```python
from build123d import *

# Parameters (mm, degrees)
SKETCH1_W                      = 6
SKETCH1_H                      = 27
BOSS_EXTRUDE1_DEPTH            = 5
BOSS_EXTRUDE2_START            = 5
BOSS_EXTRUDE2_DEPTH            = 55
CHAMFER1_SIZE                  = 20
CHAMFER1_SIZE_2                = 27.527638409
M3_CLEARANCE_HOLE1_D           = 3.6
M3_CLEARANCE_HOLE1_CSINK_D     = 3.65
M3_CLEARANCE_HOLE1_CSINK_ANGLE = 90
CUT_EXTRUDE1_DEPTH             = 70.865943062
CUT_EXTRUDE1_DEPTH_BACK        = 70.865943062
SKETCH4_R                      = 6.5
F_5_3_5_3_DIAMETER_HOLE1_D     = 5.3
F_5_3_5_3_DIAMETER_HOLE1_DEPTH = 7
F_5_3_5_3_DIAMETER_HOLE1_TIP   = 1.59228064
SKETCH10_R                     = 3
CUT_EXTRUDE2_DEPTH             = 10
SKETCH11_R                     = 2.5
CUT_EXTRUDE3_DEPTH             = 81.857900047


with BuildPart() as part:
    # Sketch1 → Boss-Extrude1 (new body)
    with BuildSketch(Plane(origin=(0, 0, 0), x_dir=(1, 0, 0), z_dir=(0, 1, 0))):
        with Locations((-20.5, -13.5)):
            Rectangle(SKETCH1_W, SKETCH1_H)
        Polygon((-23.5, 0), (-17.5, 0), (17.5, 0), (23.5, 0), (23.5, 6), (-23.5, 6), align=None)
        with Locations((20.5, -13.5)):
            Rectangle(SKETCH1_W, SKETCH1_H)
    extrude(amount=BOSS_EXTRUDE1_DEPTH)

    # Sketch1<3> → Boss-Extrude2 (add)
    with BuildSketch(Plane(origin=(0, 0, 0), x_dir=(1, 0, 0), z_dir=(0, 1, 0)).offset(BOSS_EXTRUDE2_START)):
        Polygon((-23.5, 0), (-17.5, 0), (17.5, 0), (23.5, 0), (23.5, 6), (-23.5, 6), align=None)
    extrude(amount=BOSS_EXTRUDE2_DEPTH)

    # Chamfer1
    # the kernel refuses this chamfer: 27.527638409, 20 mm, written as the material it adds along each edge
    with BuildSketch(Plane(origin=(-53.564551252, 5, 0), x_dir=(0, 0.9990705747005859, -0.043104370630376254), z_dir=(1, 0, 0))) as chamfer1_piece_1_section:
        Polygon((CHAMFER1_SIZE * 0.999070574701, CHAMFER1_SIZE * 0.0431043706304), (-CHAMFER1_SIZE_2 * 0.043104370631, CHAMFER1_SIZE_2 * 0.999070574716), (0, 0), align=None)
    chamfer1_piece_1 = extrude(amount=77.064551252, mode=Mode.PRIVATE)
    chamfer1_piece_1 = split(chamfer1_piece_1, bisect_by=Plane(origin=(-23.5, 11.537219217, 9.073559483), z_dir=(1, 0, 0)), keep=Keep.TOP, mode=Mode.PRIVATE)
    chamfer1_piece_1 = split(chamfer1_piece_1, bisect_by=Plane(origin=(-17.5, 11.537219217, 9.073559483), z_dir=(-1, 0, 0)), keep=Keep.TOP, mode=Mode.PRIVATE)
    chamfer1_piece_1 = split(chamfer1_piece_1, bisect_by=Plane(origin=(-20.5, 11.537219217, 27), z_dir=(0, 0, -1)), keep=Keep.TOP, mode=Mode.PRIVATE)
    add(chamfer1_piece_1)
    with BuildSketch(Plane(origin=(17.5, 5, 0), x_dir=(0, 0.9990705747005859, -0.04310437063037649), z_dir=(1, 0, 0))) as chamfer1_piece_2_section:
        Polygon((CHAMFER1_SIZE * 0.999070574701, CHAMFER1_SIZE * 0.0431043706304), (-CHAMFER1_SIZE_2 * 0.043104370631, CHAMFER1_SIZE_2 * 0.999070574716), (0, 0), align=None)
    chamfer1_piece_2 = extrude(amount=6, mode=Mode.PRIVATE)
    chamfer1_piece_2 = split(chamfer1_piece_2, bisect_by=Plane(origin=(20.5, 11.537219217, 27), z_dir=(0, 0, -1)), keep=Keep.TOP, mode=Mode.PRIVATE)
    add(chamfer1_piece_2)
    with BuildSketch(Plane(origin=(-23.5, 5, 0), x_dir=(0, -0.022768510603911572, 0.9997407638607518), z_dir=(1, 0, 0))) as chamfer1_piece_3_section:
        Polygon((CHAMFER1_SIZE_2 * 0.999740763876, -CHAMFER1_SIZE_2 * 0.0227685106043), (-CHAMFER1_SIZE * 0.0227685106039, -CHAMFER1_SIZE * 0.999740763861), (0, 0), align=None)
    chamfer1_piece_3 = extrude(amount=6, mode=Mode.PRIVATE)
    chamfer1_piece_3 = split(chamfer1_piece_3, bisect_by=Plane(origin=(-20.5, 11.537219217, 27), z_dir=(0, 0, -1)), keep=Keep.TOP, mode=Mode.PRIVATE)
    add(chamfer1_piece_3)
    with BuildSketch(Plane(origin=(-23.5, 5, 0), x_dir=(0, -0.022768510603911572, 0.9997407638607518), z_dir=(1, 0, 0))) as chamfer1_piece_4_section:
        Polygon((CHAMFER1_SIZE_2 * 0.999740763876, -CHAMFER1_SIZE_2 * 0.0227685106043), (-CHAMFER1_SIZE * 0.0227685106039, -CHAMFER1_SIZE * 0.999740763861), (0, 0), align=None)
    chamfer1_piece_4 = extrude(amount=77.064551252, mode=Mode.PRIVATE)
    chamfer1_piece_4 = split(chamfer1_piece_4, bisect_by=Plane(origin=(20.5, 11.537219217, 27), z_dir=(0, 0, -1)), keep=Keep.TOP, mode=Mode.PRIVATE)
    chamfer1_piece_4 = split(chamfer1_piece_4, bisect_by=Plane(origin=(23.5, 11.537219217, 9.073559483), z_dir=(-1, 0, 0)), keep=Keep.TOP, mode=Mode.PRIVATE)
    chamfer1_piece_4 = split(chamfer1_piece_4, bisect_by=Plane(origin=(17.5, 11.537219217, 9.073559483), z_dir=(1, 0, 0)), keep=Keep.TOP, mode=Mode.PRIVATE)
    add(chamfer1_piece_4)

    # M3 Clearance Hole1 (through all)
    with Locations(Plane.XY):
        with Locations((8.5, 56.5), (19.325317547, 50.25), (19.325317547, 37.75), (8.5, 31.5), (-2.325317547, 37.75), (-2.325317547, 50.25)):
            CounterSinkHole(M3_CLEARANCE_HOLE1_D / 2, M3_CLEARANCE_HOLE1_CSINK_D / 2, counter_sink_angle=M3_CLEARANCE_HOLE1_CSINK_ANGLE)

    # Sketch4 → Cut-Extrude1 (cut, two sides: drawn at the far end of the back side and taken through both)
    with BuildSketch(Plane.XY.offset(-CUT_EXTRUDE1_DEPTH_BACK)):
        with Locations((8.5, 44)):
            Circle(SKETCH4_R)
    extrude(amount=CUT_EXTRUDE1_DEPTH + CUT_EXTRUDE1_DEPTH_BACK, mode=Mode.SUBTRACT)

    # Ø5.3 (5.3) Diameter Hole1
    with Locations(Plane(origin=(0, 0, 0), x_dir=(-1, 0, 0), z_dir=(0, -1, 0))):
        with Locations((-20.5, 3), (-20.5, -15), (20.5, 3), (20.5, -15)):
            Hole(F_5_3_5_3_DIAMETER_HOLE1_D / 2, depth=F_5_3_5_3_DIAMETER_HOLE1_DEPTH)
            with Locations((0, 0, -(F_5_3_5_3_DIAMETER_HOLE1_DEPTH + F_5_3_5_3_DIAMETER_HOLE1_TIP / 2))):  # 118° drill point
                Cone(0, F_5_3_5_3_DIAMETER_HOLE1_D / 2, F_5_3_5_3_DIAMETER_HOLE1_TIP, mode=Mode.SUBTRACT)

    # Sketch10 → Cut-Extrude2 (cut)
    with BuildSketch(Plane.XY):
        with Locations((0, 23.5)):
            Circle(SKETCH10_R)
    extrude(amount=-CUT_EXTRUDE2_DEPTH, mode=Mode.SUBTRACT)

    # Sketch11 → Cut-Extrude3 (cut, through all)
    with BuildSketch(Plane.ZY.offset(23.5)):
        with Locations((5, 6)):
            Circle(SKETCH11_R)
    extrude(amount=-CUT_EXTRUDE3_DEPTH, mode=Mode.SUBTRACT)


solid = part.part
```
Verification items for the finished model (mm, model axes). A direction names the side the tool comes from. Give positions to 0.01 mm unless a question says otherwise; leave off trailing zeros. Loops run counter-clockwise (first coordinate to the right, second up) from the corner with the lowest first, then second, coordinate; pieces in that order, holes last. Notation, with made-up numbers: M -4,-37.75 L 21,-37.75 A9 cw 21,-24.75 Z; hole C 43.5,76.5 d3. An arc over 180 degrees is marked long. One line per question, with ' | ' between items.
Item 1: Section check C-C, the plane z = 6. Record the cut outline in (x, y).
Completed:
outline: M -23.5,0 L -17.5,0 L -17.5,3.71 L -23.5,3.71 Z; M -23.5,8.29 L -17.5,8.29 L -17.5,20.64 L -23.5,20.64 Z; M 17.5,0 L 23.5,0 L 23.5,3.71 L 17.5,3.71 Z; M 17.5,8.29 L 23.5,8.29 L 23.5,20.64 L 17.5,20.64 Z
Item 2: Thickness scan on line 1 (Z direction, x = -20.5, y = 2.75); line 2 (Y direction, x = 8.5, z = -1.8); line 3 (Y direction, x = 0, z = -1). Record the ranges inside material, lowest first. Write a range as [from, to].
Completed:
line 1: z = [-6, -5.65], [-0.35, 12.35], [17.65, 27] | line 2: y = [0, 29.7], [33.3, 37.5], [50.5, 54.7], [58.3, 60] | line 3: y = [0, 20.5], [26.5, 60]
Item 3: Section check D-D, the plane y = 44. Record the cut outline in (x, z).
Completed:
outline: M -23.5,-6 L 2,-6 L 2,0 L -23.5,0 Z; M 15,-6 L 23.5,-6 L 23.5,0 L 15,0 Z
Item 4: Depth check by flat-ended pin: P1, Ø6, axis at x = -7, y = 17, coming from the +Z side. Enter the tip coordinate at first touch or a pass-through.
Completed:
P1: stops at z = 0
Item 5: Draft check along Y on faces 1 (the face through (-23.5, 16, 3)), 2 (the face through (-20.939, 8.316, -3.138)), 3 (the face through (-20.542, 6.751, 7.385)). Enter one of: +Y half, -Y half, draft (parallel to the pull), parting line (faces both ways), or undercut.
Completed:
face 1: draft | face 2: -Y half | face 3: undercut
Item 6: Section check A-A, the plane y = 56.5. Record the cut outline in (x, z) (3 decimals), plus the area to 3 significant figures.
Completed:
outline: M -23.5,-6 L 6.7,-6 L 6.7,-0.025 L 6.675,0 L -23.5,0 Z; M 10.3,-6 L 23.5,-6 L 23.5,0 L 10.325,0 L 10.3,-0.025 Z | area: 260 mm^2
Item 7: Section check B-B, the plane x = 8.5. Record the cut outline in (y, z) (3 decimals), plus the area to 3 significant figures.
Completed:
outline: M 0,-6 L 29.7,-6 L 29.7,-0.025 L 29.675,0 L 0,0 Z; M 33.3,-6 L 37.5,-6 L 37.5,0 L 33.325,0 L 33.3,-0.025 Z; M 50.5,-6 L 54.7,-6 L 54.7,-0.025 L 54.675,0 L 50.5,0 Z; M 58.3,-6 L 60,-6 L 60,0 L 58.325,0 L 58.3,-0.025 Z | area: 239 mm^2
Item 8: Tool access check on faces 4 (the face through (19.56, 52.035, -3.054)), 5 (the face through (17.5, 9, 10)), 6 (the face through (0, 30, 0)). Record the directions out of +Z, -Z, +X, -X, +Y, -Y that give a thin tool (end or side, any length) a straight path to the whole face; none if there is none.
Completed:
face 4: +Z, -Z | face 5: +Z, +Y, -Y | face 6: +Z, +Y
